from build123d import *

# Parameters (mm, degrees)
F0_R     = 13
F1_DEPTH = 30
F2_W     = 55
F2_H     = 50
F3_DEPTH = 5
F5_DEPTH = 15
F6_W     = 12.6459868625
F6_H     = 18.7160577625
F7_DEPTH = 10


with BuildPart() as f1:
    # F0 (on Right) → F1 (new body)
    with BuildSketch(Plane.YZ):
        with BuildLine():
            Line((0, 50), (0, 0))
            Line((0, 0), (55, 0))
            Line((55, 0), (55, -25))
            Line((55, -25), (80, -25))
            Line((80, -25), (80, 0))
            ThreePointArc((80, 0), (82.9289321881, 7.0710678119), (90, 10))
            Line((90, 10), (110, 10))
            ThreePointArc((110, 10), (117.0710678119, 7.0710678119), (120, 0))
            Line((120, 0), (120, -40))
            Line((120, -40), (135, -40))
            Line((135, -40), (135, 0))
            Line((135, 0), (145, 0))
            Line((145, 0), (145, 70))
            Line((145, 70), (115, 70))
            Line((115, 70), (115, 30))
            Line((115, 30), (90, 30))
            Line((90, 30), (90, 90))
            Line((90, 90), (60, 90))
            Line((60, 90), (60, 50))
            Line((60, 50), (0, 50))
        make_face()
        with Locations((30, 25)):
            Circle(F0_R, mode=Mode.SUBTRACT)
    extrude(amount=F1_DEPTH)

    # F2 (on face) → F3 (join)
    with BuildSketch(Plane.YZ.offset(30)):
        with Locations((27.5, 25)):
            Rectangle(F2_W, F2_H)
    extrude(amount=-F3_DEPTH)

    # F4 (on face) → F5 (cut)
    with BuildSketch(Plane.XZ):
        with BuildLine():
            Line((13, 26.0717967697), (13, 21.5358983849))
            ThreePointArc((13, 21.5358983849), (15, 14.0717967697), (17, 21.5358983849))
            Line((17, 21.5358983849), (17, 26.0717967697))
            ThreePointArc((17, 26.0717967697), (16.4142135624, 27.4860103321), (15, 28.0717967697))
            ThreePointArc((15, 28.0717967697), (13.5857864376, 27.4860103321), (13, 26.0717967697))
        make_face()
    extrude(amount=-F5_DEPTH, mode=Mode.SUBTRACT)

    # F6 (on face) → F7 (cut)
    with BuildSketch(Plane.XZ.offset(-15)):
        with Locations((15.175185632, 21.5370440856)):
            Rectangle(F6_W, F6_H)
    extrude(amount=F7_DEPTH, mode=Mode.SUBTRACT)


solid = f1.part
Can you work these out from the model? Positions are in its coordinate system, mm. A direction names the side the tool comes from. Give positions to 0.01 mm unless a question says otherwise; leave off trailing zeros. Loops run counter-clockwise (first coordinate to the right, second up) from the corner with the lowest first, then second, coordinate; pieces in that order, holes last. Notation, with made-up numbers: (77, 51) - (129, 51) arc R29 cw to (129, 87) - close; hole circle Ø4 at (-10.5, -24). An arc over 180 degrees is marked (long way). Answer as a JSON object with one key per item and string values.
Q1. Imagine slicing it at A-A on z = -16. Write out the boundary of the cut face in (x, y), plus the area to 3 significant figures.
Geometry says:
{"outline": "(0, 55) - (30, 55) - (30, 80) - (0, 80) - close; (0, 120) - (30, 120) - (30, 135) - (0, 135) - close", "area": "1,200 mm²"}
Q2. Will these pins go through, and if not, where does the flat tip stop? P1, Ø4, axis at x = 4, z = -24, coming from the -Y side; P2, Ø8, axis at x = 18.5, y = 142.5, coming from the -Z side; P3, Ø9, axis at x = 15, z = 18.07, coming from the -Y side; P4, Ø7.5, axis at x = 20.5, y = 70, coming from the -Z side.
Geometry says:
{"P1": "y = 55", "P2": "z = 0", "P3": "y = 0", "P4": "z = -25"}
Q3. If we mould it in two halves opening along X, with no side actions, what happens to faces 1 (the flat face through (30, 71, 26)), 2 (the flat face through (15, 10, 12.179)), 3 (the flat face through (15, 100, 10))? For each: pulls with the +X half, pulls with the -X half, needs draft (parallel to the pull), parting line crosses it, or undercut.
Geometry says:
{"face 1": "pulls with the +X half", "face 2": "undercut", "face 3": "needs draft"}
Q4. If I drill on L1, parallel to Z at x = 8.25, y = 30; L2, parallel to Y at x = 14, z = 25; L3, parallel to Y at x = 24.5, z = 65.5, over which ranges is the centre line in solid material (lowest first)?
Geometry says:
{"L1": "0 to 12, 38 to 50", "L2": "15 to 17, 43 to 145", "L3": "60 to 90, 115 to 145"}
Q5. Imagine slicing it at B-B on x = 6.25. Write out the boundary of the cut face in (y, z), plus the area to 3 significant figures.
Geometry says:
{"outline": "(0, 0) - (55, 0) - (55, -25) - (80, -25) - (80, 0) arc R10 cw to (90, 10) - (110, 10) arc R10 cw to (120, 0) - (120, -40) - (135, -40) - (135, 0) - (145, 0) - (145, 70) - (115, 70) - (115, 30) - (90, 30) - (90, 90) - (60, 90) - (60, 50) - (0, 50) - close; hole circle Ø26 at (30, 25)", "area": "8,890 mm²"}
Q6. Imagine slicing it at C-C on y = 10.5. Write out the boundary of the cut face in (x, z), plus the area to 3 significant figures.
Geometry says:
{"outline": "(0, 0) - (30, 0) - (30, 50) - (0, 50) - close; hole (8.85, 12.18) - (21.5, 12.18) - (21.5, 30.9) - (8.85, 30.9) - close", "area": "1,260 mm²"}
Q7. Imagine slicing it at D-D on y = 30. Write out the boundary of the cut face in (x, z).
Geometry says:
{"outline": "(0, 0) - (30, 0) - (30, 50) - (0, 50) - (0, 38) - (25, 38) - (25, 12) - (0, 12) - close"}
Q8. Which directions (+Z, -Z, +X, -X, +Y, -Y) give clear straight access to the entire face, cutting with the end or side of a thin tool? Please do faces 4 (the flat face through (15, 27, 0)), 5 (the cylindrical face through (12.325, 17.013, 25.572)), 6 (the flat face through (21.498, 10, 21)), 7 (the flat face through (15, 30, 50)), 8 (the cylindrical face through (14.853, 2.465, 14.074)).
Geometry says:
{"face 4": "-Z, +X, -X, -Y", "face 5": "-X", "face 6": "none", "face 7": "+Z, +X, -X, -Y", "face 8": "-Y"}
